Design review of the part built by this model. Coordinates are the model's own, in mm. A direction names the side the tool comes from. Coordinates: 2 decimals unless noted, no trailing zeros. Write each loop counter-clockwise with the first axis right and the second up, starting at its lowest first coordinate (ties: lowest second). Pieces come first, ordered by that corner, then holes. Notation, with made-up numbers: (8, 70.5) - (50, 70.5) arc R16 ccw to (50, 81.5) - close; hole circle Ø4 at (43.5, -28). An arc over 180 degrees is marked (long way). Answer as a JSON object with one key per item and string values.
```python
from build123d import *

# Parameters (mm, degrees)
SKETCH1_R                   = 16
BOSS_EXTRUDE1_DEPTH         = 2.5
TAP_DRILL_FOR_M4X0_7_TAP1_D = 3.3


with BuildPart() as part:
    # Sketch1 → Boss-Extrude1 (new body, symmetric)
    with BuildSketch(Plane.XY):
        Circle(SKETCH1_R)
        with BuildLine():
            Line((-2.5, 4.387767086), (2.5, 4.387767086))
            ThreePointArc((2.5, 4.387767086), (0, -5.05), (-2.5, 4.387767086))
        make_face(mode=Mode.SUBTRACT)
    extrude(amount=BOSS_EXTRUDE1_DEPTH, both=True)

    # Tap Drill for M4x0.7 Tap1 (through all)
    with Locations(Plane.XY.offset(2.5)):
        with Locations((8.485281374, 8.485281374), (-8.485281374, 8.485281374), (-8.485281374, -8.485281374), (8.485281374, -8.485281374)):
            Hole(TAP_DRILL_FOR_M4X0_7_TAP1_D / 2)


solid = part.part
```
(1) To check wall thickness, follow line 1 (Y direction, x = 9, z = -2.2); line 2 (Y direction, x = 7, z = 2.3); line 3 (X direction, y = 9.5, z = 1.05). State the ranges of each line that lie inside material, in increasing order. Write a range as from..to.
Solved:
{"line 1": "y = -13.23..-10.05, -6.92..6.92, 10.05..13.23", "line 2": "y = -14.39..-9.2, -7.77..7.77, 9.2..14.39", "line 3": "x = -12.87..-9.79, -7.18..7.18, 9.79..12.87"}
(2) Take a section at D-D, the plane z = 0.35. Write out the cut boundary in (x, y), and give its area (3 significant figures).
Solved:
{"outline": "circle Ø32 at (0, 0); hole circle Ø3.3 at (-8.49, -8.49); hole circle Ø3.3 at (-8.49, 8.49); hole (-2.5, 4.39) arc R5.05 ccw (long way) to (2.5, 4.39) - close; hole circle Ø3.3 at (8.49, -8.49); hole circle Ø3.3 at (8.49, 8.49)", "area": "692 mm^2"}
(3) The part is to be moulded in two halves that separate along Y. For faces 3 (the face through (-4, 4, 2.5)), 4 (the face through (-3.47, -15.62, 0.04)), 5 (the face through (10.134, -8.413, -0.035)), say which applies: pulls with the +Y half, pulls with the -Y half, needs draft (parallel to the pull), parting line crosses it, or undercut.
Solved:
{"face 3": "needs draft", "face 4": "parting line crosses it", "face 5": "undercut"}
(4) Take a section at A-A, the plane y = 0. Write out the cut boundary in (x, z).
Solved:
{"outline": "(-16, -2.5) - (-5.05, -2.5) - (-5.05, 2.5) - (-16, 2.5) - close; (5.05, -2.5) - (16, -2.5) - (16, 2.5) - (5.05, 2.5) - close"}
(5) Tool access review of faces 1 (the face through (-4, 4, -2.5)), 2 (the face through (0, 4.388, 0)): name each direction out of +Z, -Z, +X, -X, +Y, -Y from which nothing blocks a thin tool from reaching the whole face with its end or side.
Solved:
{"face 1": "-Z, +X, -X, +Y, -Y", "face 2": "+Z, -Z"}
(6) Take a section at B-B, the plane x = 0. Write out the cut boundary in (y, z), and give its area (3 significant figures).
Solved:
{"outline": "(-16, -2.5) - (-5.05, -2.5) - (-5.05, 2.5) - (-16, 2.5) - close; (4.39, -2.5) - (16, -2.5) - (16, 2.5) - (4.39, 2.5) - close", "area": "113 mm^2"}
(7) For pin 1 (1 mm diameter, centred on x = -9, z = 1, fed in from +Y); pin 2 (3 mm diameter, centred on x = -10.5, z = 0.5, fed in from -Y); pin 3 (1 mm diameter, centred on y = 6, z = -0.5, fed in from -X) (3 decimals), all flat-tipped, find the tip position at first contact; note any pin that passes through.
Solved:
{"pin 1": "stops at y = 13.56", "pin 2": "stops at y = -13.23", "pin 3": "stops at x = -15.025"}
(8) Take a section at C-C, the plane y = 7.5. Write out the cut boundary in (x, z).
Solved:
{"outline": "(-14.13, -2.5) - (-9.81, -2.5) - (-9.81, 2.5) - (-14.13, 2.5) - close; (-7.16, -2.5) - (7.16, -2.5) - (7.16, 2.5) - (-7.16, 2.5) - close; (9.81, -2.5) - (14.13, -2.5) - (14.13, 2.5) - (9.81, 2.5) - close"}
